from build123d import *

# Parameters (mm, degrees)
F1_DEPTH  = 18.5547
F3_DEPTH  = 33.9344
F4_W      = 45.72
F4_H      = 45.72
F5_DEPTH  = 6.35
F6_R      = 1.5875
F7_DEPTH  = 4.7752
F8_R      = 1.5875
F9_W      = 6.35
F9_H      = 0.762
F10_DEPTH = 27.5844
F11_SIZE  = 1.27


with BuildPart() as f1:
    # F0 (on Top) → F1 (new body, symmetric)
    with BuildSketch(Plane.XY):
        with BuildLine():
            ThreePointArc((24.1935, 22.606), (23.7285320151, 23.7285320151), (22.606, 24.1935))
            Line((22.606, 24.1935), (-22.606, 24.1935))
            ThreePointArc((-22.606, 24.1935), (-23.7285320151, 23.7285320151), (-24.1935, 22.606))
            Line((-24.1935, 22.606), (-24.1935, -22.606))
            ThreePointArc((-24.1935, -22.606), (-23.7285320151, -23.7285320151), (-22.606, -24.1935))
            Line((-22.606, -24.1935), (22.606, -24.1935))
            ThreePointArc((22.606, -24.1935), (23.7285320151, -23.7285320151), (24.1935, -22.606))
            Line((24.1935, -22.606), (24.1935, 22.606))
        make_face()
    extrude(amount=F1_DEPTH, both=True)

    # F2 (on face) → F3 (cut)
    with BuildSketch(Plane.XY.offset(18.5547)):
        Polygon((20.828, -20.3835), (20.828, 20.3835), (20.828, 20.828), (20.3835, 20.828), (-20.3835, 20.828), (-20.828, 20.828), (-20.828, 20.3835), (-20.828, -20.3835), (-20.828, -20.828), (-20.3835, -20.828), (20.3835, -20.828), (20.828, -20.828), align=None)
    extrude(amount=-F3_DEPTH, mode=Mode.SUBTRACT)

    # F4 (on face) → F5 (cut)
    with BuildSketch(Plane.XY.offset(18.5547)):
        Rectangle(F4_W, F4_H)
    extrude(amount=-F5_DEPTH, mode=Mode.SUBTRACT)

    # F6 (on face) → F7 (join)
    with BuildSketch(Plane.XY.offset(-15.3797)):
        with Locations((17.4514236985, -17.4514236985)):
            Circle(F6_R)
        with Locations((-17.4514236985, -17.4514236985)):
            Circle(F6_R)
        with Locations((-17.4514236985, 17.4514236985)):
            Circle(F6_R)
        with Locations((17.4514236985, 17.4514236985)):
            Circle(F6_R)
    extrude(amount=F7_DEPTH)

    # F8
    f8_edges = [f1.edges().sort_by_distance(p)[0] for p in [
        (22.86, 22.86, 15.3797),
        (-22.86, 22.86, 15.3797),
        (-22.86, -22.86, 15.3797),
        (22.86, -22.86, 15.3797),
    ]]
    fillet(f8_edges, radius=F8_R)

    # F9 (on face) → F10 (cut, through all)
    with BuildSketch(Plane.XY.offset(12.2047)):
        with Locations((0, 21.209)):
            Rectangle(F9_W, F9_H)
        with Locations((0, -21.209)):
            Rectangle(F9_W, F9_H)
    extrude(amount=-F10_DEPTH, mode=Mode.SUBTRACT)

    # F11
    f11_edges = [f1.edges().sort_by_distance(p)[0] for p in [
        (-23.728532, 23.728532, 18.5547),
        (-24.1935, 0, 18.5547),
        (-23.728532, -23.728532, 18.5547),
        (0, -24.1935, 18.5547),
        (23.728532, -23.728532, 18.5547),
        (24.1935, 0, 18.5547),
        (0, 24.1935, 18.5547),
    ]]
    chamfer(f11_edges, length=F11_SIZE)


solid = f1.part
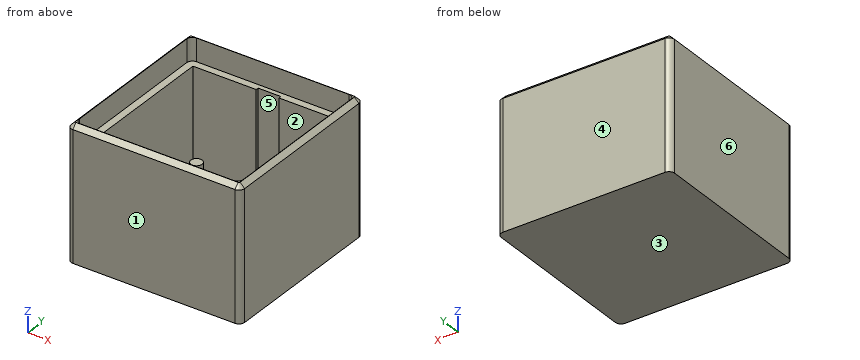
Geometry check sheet. Reference: the model listing, model coordinates, mm. Face numbers are marked on the shaded views. A direction names the side the tool comes from. Give positions to 0.01 mm unless a question says otherwise; leave off trailing zeros. Write each loop counter-clockwise with the first axis right and the second up, starting at its lowest first coordinate (ties: lowest second). Pieces come first, ordered by that corner, then holes.
1) Release check for a two-part mould opening along Y. For the marked faces 1, 2, 3 and 4 record: released by +Y, released by -Y, zero draft, split by the parting line, or undercut.
Values follow:
face 1: released by -Y
face 2: undercut
face 3: zero draft
face 4: released by +Y
2) Cross-section at B-B (z = 13.5). Record the boundary of the cut face in (x, y) (1 decimal), plus the area to 3 significant figures.
Values follow:
outline: (-24.2, -22.6) arc R1.6 ccw to (-22.6, -24.2) - (22.6, -24.2) arc R1.6 ccw to (24.2, -22.6) - (24.2, 22.6) arc R1.6 ccw to (22.6, 24.2) - (-22.6, 24.2) arc R1.6 ccw to (-24.2, 22.6) - close; hole (-22.9, -21.3) arc R1.6 ccw to (-21.3, -22.9) - (21.3, -22.9) arc R1.6 ccw to (22.9, -21.3) - (22.9, 21.3) arc R1.6 ccw to (21.3, 22.9) - (-21.3, 22.9) arc R1.6 ccw to (-22.9, 21.3) - close
area: 251 mm2
3) Set-up check for the marked faces 5 and 6: record each of +Z, -Z, +X, -X, +Y, -Y from which the full face is reachable in a straight line by a thin tool's end or side.
Values follow:
face 5: +Z
face 6: +Z, -Z, -X, +Y, -Y
4) Cross-section at A-A (x = -2.5). Record the boundary of the cut face in (y, z).
Values follow:
outline: (-24.19, -18.55) - (24.19, -18.55) - (24.19, 17.28) - (22.92, 18.55) - (22.86, 18.55) - (22.86, 12.2) - (21.59, 12.2) - (21.59, -15.38) - (-21.59, -15.38) - (-21.59, 12.2) - (-22.86, 12.2) - (-22.86, 18.55) - (-22.92, 18.55) - (-24.19, 17.28) - close
5) Thickness scan on line 1 (X direction, y = -16.5, z = 3.5); line 2 (Y direction, x = 3, z = 3.5). Record the ranges inside material, lowest first.
Values follow:
line 1: x = -24.19 to -20.83, 20.83 to 24.19
line 2: y = -24.19 to -21.59, 21.59 to 24.19
6) Cross-section at C-C (y = 0.5). Record the boundary of the cut face in (x, z), plus the area to 3 significant figures.
Values follow:
outline: (-24.19, -18.55) - (24.19, -18.55) - (24.19, 17.28) - (22.92, 18.55) - (22.86, 18.55) - (22.86, 12.2) - (20.83, 12.2) - (20.83, -15.38) - (-20.83, -15.38) - (-20.83, 12.2) - (-22.86, 12.2) - (-22.86, 18.55) - (-22.92, 18.55) - (-24.19, 17.28) - close
area: 355 mm2
7) Go/stop test with flat-tipped pins: pin 1 Ø1.6 at (x, y) = (18, -18) entering from +Z; pin 2 Ø8 at (x, y) = (0.5, -11.5) entering from +Z. Record where each tip stops, or that it passes through.
Values follow:
pin 1: stops at z = -10.6
pin 2: stops at z = -15.38
8) Cross-section at D-D (z = -2). Record the boundary of the cut face in (x, y) (1 decimal), plus the area to 3 significant figures.
Values follow:
outline: (-24.2, -22.6) arc R1.6 ccw to (-22.6, -24.2) - (22.6, -24.2) arc R1.6 ccw to (24.2, -22.6) - (24.2, 22.6) arc R1.6 ccw to (22.6, 24.2) - (-22.6, 24.2) arc R1.6 ccw to (-24.2, 22.6) - close; hole (-20.8, -20.8) - (-3.2, -20.8) - (-3.2, -21.6) - (3.2, -21.6) - (3.2, -20.8) - (20.8, -20.8) - (20.8, 20.8) - (3.2, 20.8) - (3.2, 21.6) - (-3.2, 21.6) - (-3.2, 20.8) - (-20.8, 20.8) - close
area: 594 mm2
